Can you work these out from the model? Positions are in its coordinate system, mm. Give positions to 0.01 mm unless a question says otherwise; leave off trailing zeros. Order: outer loops, then holes, each group sorted by start corner. A loop starts at its lowest first (then second) coordinate and runs counter-clockwise, first axis right, second up. Notation, with made-up numbers: (41, 72.25) -> (65, 72.25) arc R6 ccw to (65, 80.25) -> close; hole circle Ø1 at (-24.5, 57). An arc over 180 degrees is marked (long way). Answer as a JSON object with one key per item and string values.
```python
from build123d import *

# Parameters (mm, degrees)
SKETCH1_R           = 1.651
BOSS_EXTRUDE1_DEPTH = 1.5875


with BuildPart() as part:
    # Sketch1 → Boss-Extrude1 (new body)
    with BuildSketch(Plane(origin=(0, 0, 0), x_dir=(-1, 0, 0), z_dir=(0, 0, -1))):
        with BuildLine():
            Line((-156.36875, 0), (-5.55625, 0))
            ThreePointArc((-5.55625, 0), (-1.627387947, 1.627387947), (0, 5.55625))
            Line((0, 5.55625), (0, 156.368750002))
            ThreePointArc((0, 156.368750002), (-1.627387947, 160.297612055), (-5.55625, 161.925000002))
            Line((-5.55625, 161.925000002), (-53.373846022, 161.925000002))
            ThreePointArc((-53.373846022, 161.925000002), (-53.971512021, 161.892762078), (-54.562242583, 161.796422402))
            Line((-54.562242583, 161.796422402), (-109.634404321, 149.738294575))
            ThreePointArc((-109.634404321, 149.738294575), (-111.112127046, 149.185426993), (-112.374869815, 148.239484227))
            Line((-112.374869815, 148.239484227), (-148.239484217, 112.374869825))
            ThreePointArc((-148.239484217, 112.374869825), (-149.185426983, 111.112127057), (-149.738294565, 109.634404332))
            Line((-149.738294565, 109.634404332), (-161.796422399, 54.562242596))
            ThreePointArc((-161.796422399, 54.562242596), (-161.892762076, 53.971512033), (-161.925, 53.373846033))
            Line((-161.925, 53.373846033), (-161.925, 5.55625))
            ThreePointArc((-161.925, 5.55625), (-160.297612053, 1.627387947), (-156.36875, 0))
        make_face()
        with Locations((-26.9875, 134.9375)):
            Circle(SKETCH1_R, mode=Mode.SUBTRACT)
        with Locations((-26.9875, 80.9625)):
            Circle(SKETCH1_R, mode=Mode.SUBTRACT)
        with Locations((-26.9875, 26.9875)):
            Circle(SKETCH1_R, mode=Mode.SUBTRACT)
        with Locations((-134.9375, 26.9875)):
            Circle(SKETCH1_R, mode=Mode.SUBTRACT)
        with Locations((-73.058044257, 73.058044257)):
            Circle(SKETCH1_R, mode=Mode.SUBTRACT)
        with Locations((-111.224132771, 111.224132771)):
            Circle(SKETCH1_R, mode=Mode.SUBTRACT)
        with Locations((-80.9625, 26.9875)):
            Circle(SKETCH1_R, mode=Mode.SUBTRACT)
    extrude(amount=-BOSS_EXTRUDE1_DEPTH)


solid = part.part
```
1. If we section it at C-C on x = 102: Please give me the cut outline in (y, z), then the cut area to 3 significant figures.
Worked answers:
{"outline": "(0, 0) -> (151.41, 0) -> (151.41, 1.59) -> (0, 1.59) -> close", "area": "240 mm²"}
2. If we section it at A-A on z = 0.55: Please give me the cut outline in (x, y) (1 decimal), then the cut area to 3 significant figures.
Worked answers:
{"outline": "(0, 5.6) arc R5.6 ccw to (5.6, 0) -> (156.4, 0) arc R5.6 ccw to (161.9, 5.6) -> (161.9, 53.4) arc R5.6 ccw to (161.8, 54.6) -> (149.7, 109.6) arc R5.6 ccw to (148.2, 112.4) -> (112.4, 148.2) arc R5.6 ccw to (109.6, 149.7) -> (54.6, 161.8) arc R5.6 ccw to (53.4, 161.9) -> (5.6, 161.9) arc R5.6 ccw to (0, 156.4) -> close; hole circle Ø3.3 at (27, 27); hole circle Ø3.3 at (27, 81); hole circle Ø3.3 at (27, 134.9); hole circle Ø3.3 at (73.1, 73.1); hole circle Ø3.3 at (81, 27); hole circle Ø3.3 at (111.2, 111.2); hole circle Ø3.3 at (134.9, 27)", "area": "23,600 mm²"}
3. If we section it at B-B on y = 127: Please give me the cut outline in (x, z), then the cut area to 3 significant figures.
Worked answers:
{"outline": "(0, 0) -> (133.61, 0) -> (133.61, 1.59) -> (0, 1.59) -> close", "area": "212 mm²"}
4. Please list where these lines run through material, in increasing order: L1, parallel to X at y = 74, z = 1.05; L2, parallel to X at y = 106, z = 0.55; L3, parallel to X at y = 84.5, z = 0.5.
Worked answers:
{"L1": "0 to 71.7, 74.41 to 157.54", "L2": "0 to 150.53", "L3": "0 to 155.24"}
